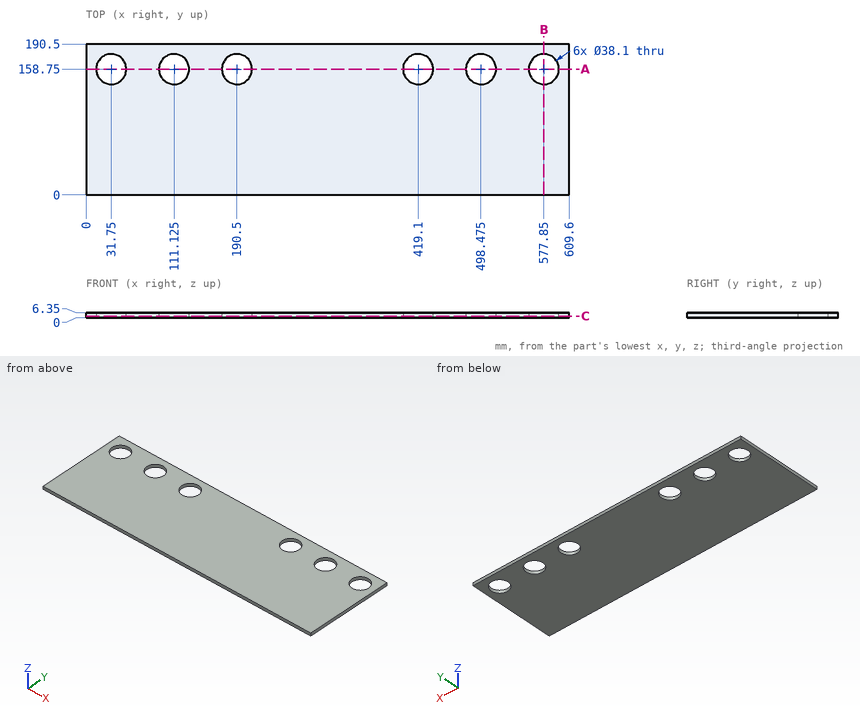
Source: three-view drawing plus pictorial views. Frame: mm from the lowest corner of the part. Round coordinates to 2 decimals unless told otherwise and drop trailing zeros. Loops run counter-clockwise (first coordinate to the right, second up) from the corner with the lowest first, then second, coordinate; pieces in that order, holes last. Notation, with made-up numbers: M -21.5,53 L -13.5,53 A11 cw -13.5,68 Z; hole C 43,-37.5 d10. An arc over 180 degrees is marked long. Put each result on its own line as item: value. Start each with the question number.
(1) Section query A-A (y = 158.75). Return loops of the section in (x, z) (3 decimals), then the cut area to 3 significant figures.
(2) Section query B-B (x = 577.85). Return loops of the section in (y, z).
(3) Material intervals for line 1 along Y through (x, z) = (577.85, 2); line 2 along Y through (x, z) = (41.5, 2), sorted ascending. Write a range as [from, to].
(4) Section query C-C (z = 2.25). Return loops of the section in (x, y) (3 decimals), then the cut area to 3 significant figures.
Findings below:
1. outline: M 0,0 L 12.7,0 L 12.7,6.35 L 0,6.35 Z; M 50.8,0 L 92.075,0 L 92.075,6.35 L 50.8,6.35 Z; M 130.175,0 L 171.45,0 L 171.45,6.35 L 130.175,6.35 Z; M 209.55,0 L 400.05,0 L 400.05,6.35 L 209.55,6.35 Z; M 438.15,0 L 479.425,0 L 479.425,6.35 L 438.15,6.35 Z; M 517.525,0 L 558.8,0 L 558.8,6.35 L 517.525,6.35 Z; M 596.9,0 L 609.6,0 L 609.6,6.35 L 596.9,6.35 Z
1. area: 2,420 mm2
2. outline: M 0,0 L 139.7,0 L 139.7,6.35 L 0,6.35 Z; M 177.8,0 L 190.5,0 L 190.5,6.35 L 177.8,6.35 Z
3. line 1: y = [0, 139.7], [177.8, 190.5]
3. line 2: y = [0, 142.38], [175.12, 190.5]
4. outline: M 0,0 L 609.6,0 L 609.6,190.5 L 0,190.5 Z; hole C 31.75,158.75 d38.1; hole C 111.125,158.75 d38.1; hole C 190.5,158.75 d38.1; hole C 419.1,158.75 d38.1; hole C 498.475,158.75 d38.1; hole C 577.85,158.75 d38.1
4. area: 109,000 mm2
